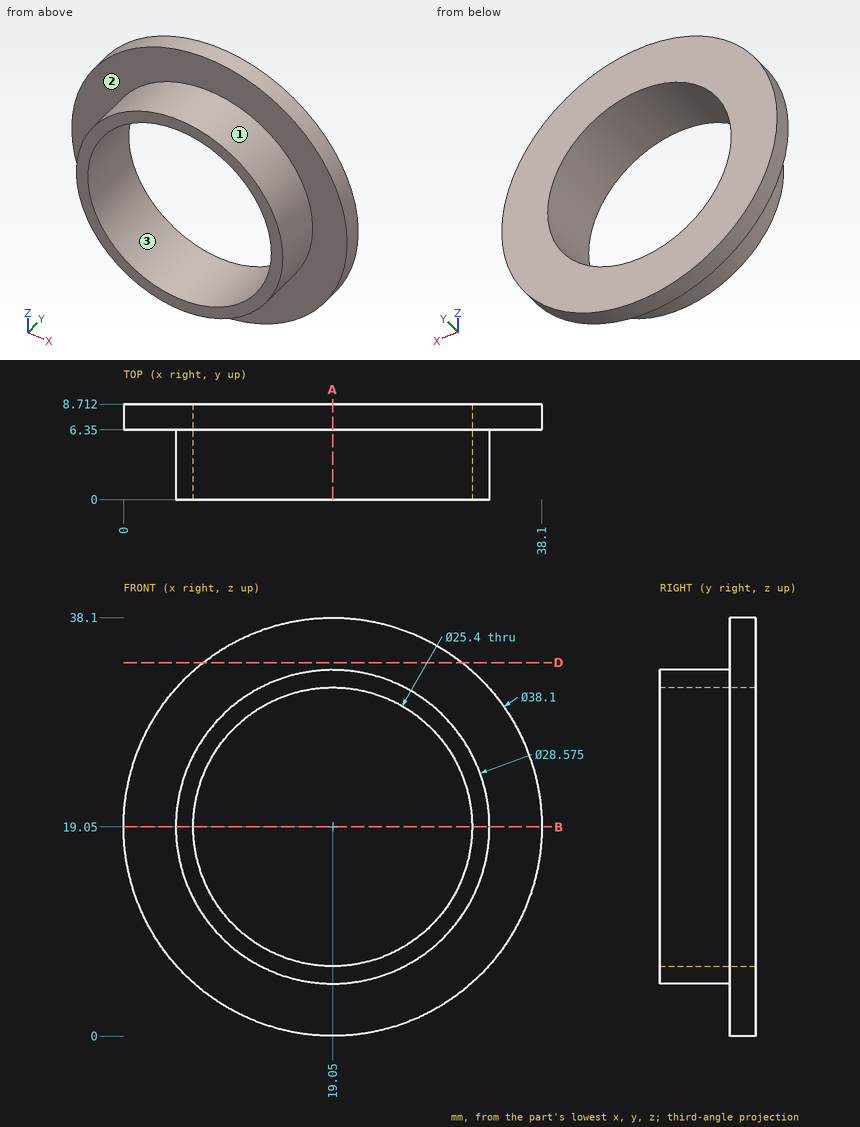
The drawing under review shows one solid part. Ordinate dimensions are in mm from its lowest x, y, z. Round coordinates to 2 decimals unless told otherwise and drop trailing zeros. Loops run counter-clockwise (first coordinate to the right, second up) from the corner with the lowest first, then second, coordinate; pieces in that order, holes last.
Item 1: Take a section at A-A (x = 19.05). Write out the cut boundary in (y, z).
Determined:
outline: (0, 4.76) - (6.35, 4.76) - (6.35, 0) - (8.71, 0) - (8.71, 6.35) - (0, 6.35) - close; (0, 31.75) - (8.71, 31.75) - (8.71, 38.1) - (6.35, 38.1) - (6.35, 33.34) - (0, 33.34) - close
Item 2: Take a section at D-D (z = 34). Write out the cut boundary in (x, y).
Determined:
outline: (7.24, 6.35) - (30.86, 6.35) - (30.86, 8.71) - (7.24, 8.71) - close
Item 3: For line 1 (Z direction, x = 19.05, y = 5.25); line 2 (Y direction, x = 6, z = 11); line 3 (X direction, y = 8, z = 9) (1 decimal), list the stretches that pass through material, from the lowest coordinate up.
Determined:
line 1: z = 4.76 to 6.35, 31.75 to 33.34
line 2: y = 6.35 to 8.71
line 3: x = 2.9 to 11.3, 26.8 to 35.2
Item 4: Mouldability with a two-part tool opening along Z and no side actions: class the marked faces 1, 2 and 3 as released by +Z, released by -Z, zero draft, split by the parting line, or undercut.
Determined:
face 1: split by the parting line
face 2: zero draft
face 3: undercut
Item 5: Clearance check with flat-ended pins moving along their axes: pin 1 Ø5 at (y, z) = (2, 7.5) entering from -X; pin 2 Ø1 at (y, z) = (3.5, 23) entering from +X (1 decimal); pin 3 Ø1.5 at (x, z) = (21, 8.5) entering from -Y; pin 4 Ø2 at (x, y) = (23, 5.5) entering from +Z. State where each tip first meets the part, or that it passes through.
Determined:
pin 1: stops at x = 7.99
pin 2: stops at x = 32.9
pin 3: passes through
pin 4: stops at z = 37.79
Item 6: Take a section at B-B (z = 19.05). Write out the cut boundary in (x, y).
Determined:
outline: (0, 6.35) - (4.76, 6.35) - (4.76, 0) - (6.35, 0) - (6.35, 8.71) - (0, 8.71) - close; (31.75, 0) - (33.34, 0) - (33.34, 6.35) - (38.1, 6.35) - (38.1, 8.71) - (31.75, 8.71) - close
